```python
from build123d import *

# Parameters (mm, degrees)
F0_R     = 2.5
F1_DEPTH = 5
F3_R     = 4.35
F4_DEPTH = 3
F5_R     = 5
F6_R     = 5
F7_R     = 1
F8_R     = 1


with BuildPart() as f1:
    # F0 (on Top) → F1 (new body)
    with BuildSketch(Plane.XY):
        with BuildLine():
            Line((0, 130), (-15, 130))
            Line((-15, 130), (-15, 70))
            ThreePointArc((-15, 70), (-31.109127, 31.109127), (-70, 15))
            Line((-70, 15), (-91.909339, 15))
            ThreePointArc((-91.909339, 15), (-108.882194, 12.237932), (-100.9, -2.993331))
            Line((-100.9, -2.993331), (-100.9, 0.560259))
            ThreePointArc((-100.9, 0.560259), (-99.4, 14.6), (-97.9, 0.560259))
            Line((-97.9, 0.560259), (-97.9, -2.993331))
            ThreePointArc((-97.9, -2.993331), (-94.662068, -1.982194), (-91.909339, 0))
            Line((-91.909339, 0), (-70, 0))
            ThreePointArc((-70, 0), (-20.502525, 20.502525), (0, 70))
            Line((0, 70), (0, 130))
        make_face()
        with Locations((-7.5, 89.3)):
            Circle(F0_R, mode=Mode.SUBTRACT)
        with Locations((-7.5, 119.8)):
            Circle(F0_R, mode=Mode.SUBTRACT)
    extrude(amount=F1_DEPTH)

    # F3 (on offset) → F4 (cut, through all)
    with BuildSketch(Plane.XY.offset(2)):
        with Locations((-7.5, 89.3)):
            Circle(F3_R)
        with Locations((-7.5, 119.8)):
            Circle(F3_R)
    extrude(amount=F4_DEPTH, mode=Mode.SUBTRACT)

    # F5
    f5_edges = [f1.edges().sort_by_distance(p)[0] for p in [
        (0, 130, 2.5),
    ]]
    fillet(f5_edges, radius=F5_R)

    # F6
    f6_edges = [f1.edges().sort_by_distance(p)[0] for p in [
        (-15, 130, 2.5),
    ]]
    fillet(f6_edges, radius=F6_R)

    # F7
    f7_edges = [f1.edges().sort_by_distance(p)[0] for p in [
        (0, 97.5, 5),
    ]]
    fillet(f7_edges, radius=F7_R)

    # F8
    f8_edges = [f1.edges().sort_by_distance(p)[0] for p in [
        (0, 97.5, 0),
    ]]
    fillet(f8_edges, radius=F8_R)


solid = f1.part
```
Geometry: final body of the model. Coordinates: model frame, mm. A direction names the side the tool comes from. Round coordinates to 2 decimals unless told otherwise and drop trailing zeros. Loops run counter-clockwise (first coordinate to the right, second up) from the corner with the lowest first, then second, coordinate; pieces in that order, holes last.
Item 1: Section D-D, the plane y = 102.5. Output: boundary loops of the cut face in (x, z), plus the area to 3 significant figures.
Checked values:
outline: (-15, 1) arc R1 ccw to (-14, 0) - (-1, 0) arc R1 ccw to (0, 1) - (0, 4) arc R1 ccw to (-1, 5) - (-14, 5) arc R1 ccw to (-15, 4) - close
area: 74.1 mm2
Item 2: Reachability of faces 5 (the flat face through (-19, 44, 0)), 6 (the flat face through (-5.6, 117.9, 2)), 7 (the flat face through (-81, 15, 2)), 8 (the flat face through (-15, 98, 2)), 9 (the cylindrical face through (-7.83, 91.78, 0.99)) from +Z, -Z, +X, -X, +Y, -Y: full face, straight path, thin tool, end or side. Return the list, or none.
Checked values:
face 5: -Z, +X, -X, +Y, -Y
face 6: +Z
face 7: +Z, -Z, +Y
face 8: +Z, -Z, -X, +Y
face 9: +Z, -Z
Item 3: Section C-C, the plane x = -76. Output: boundary loops of the cut face in (y, z), plus the area to 3 significant figures.
Checked values:
outline: (0, 1) arc R1 ccw to (1, 0) - (14, 0) arc R1 ccw to (15, 1) - (15, 4) arc R1 ccw to (14, 5) - (1, 5) arc R1 ccw to (0, 4) - close
area: 74.1 mm2
Item 4: Mould query, pull axis Y, two halves, no side actions, for faces 1 (the cylindrical face through (-21.05, 19.96, 2.48)), 2 (the cylindrical face through (-2, 129, 3)), 3 (the cylindrical face through (-5.49, 115.94, 3.48)), 4 (the cylindrical face through (-5.49, 85.44, 3.48)). Classes: released by +Y, released by -Y, zero draft, split by the parting line, or undercut.
Checked values:
face 1: released by -Y
face 2: released by +Y
face 3: undercut
face 4: undercut
Item 5: Section B-B, the plane z = 3. Output: boundary loops of the cut face in (x, y).
Checked values:
outline: (-100.9, -2.99) - (-100.9, 0.56) arc R7.1 cw (long way) to (-97.9, 0.56) - (-97.9, -2.99) arc R10.6 ccw to (-91.91, 0) - (-70, 0) arc R70 ccw to (0, 70) - (0, 125) arc R5 ccw to (-5, 130) - (-10, 130) arc R5 ccw to (-15, 125) - (-15, 70) arc R55 cw to (-70, 15) - (-91.91, 15) arc R10.6 ccw (long way) to start; hole circle Ø8.7 at (-7.5, 89.3); hole circle Ø8.7 at (-7.5, 119.8)
Item 6: Section A-A, the plane y = 119.8. Output: boundary loops of the cut face in (x, z), plus the area to 3 significant figures.
Checked values:
outline: (-15, 1) arc R1 ccw to (-14, 0) - (-10, 0) - (-10, 2) - (-11.85, 2) - (-11.85, 5) - (-14, 5) arc R1 ccw to (-15, 4) - close; (-5, 0) - (-1, 0) arc R1 ccw to (0, 1) - (0, 4) arc R1 ccw to (-1, 5) - (-3.15, 5) - (-3.15, 2) - (-5, 2) - close
area: 38.0 mm2
Item 7: Contact query for flat-ended pins moving along their axis: P1, Ø8, axis at x = -7.5, y = 119.8, coming from the -Z side; P2, Ø1.5, axis at y = 59, z = 1.5, coming from the +X side; P3, Ø1.1, axis at y = -2, z = 3.5, coming from the -X side; P4, Ø1, axis at y = 69, z = 1.5, coming from the -X side. Output: stop coordinate, or through.
Checked values:
P1: stops at z = 0
P2: stops at x = -0.75
P3: stops at x = -105.08
P4: stops at x = -15.02
Item 8: Line query: L1, parallel to X at y = 119.8, z = 1.1; L2, parallel to Y at x = -7.5, z = 0.85; L3, parallel to Y at x = -99.4, z = 1.1. Output: solid intervals per line, ascending.
Checked values:
L1: x = -15 to -10, -5 to 0
L2: y = 38.5 to 86.8, 91.8 to 117.3, 122.3 to 129.99
L3: y = 14.6 to 18.1
